Input: part model. Units: mm. Frame: model coordinates. A direction names the side the tool comes from. Coordinates: 2 decimals unless noted, no trailing zeros. Write each loop counter-clockwise with the first axis right and the second up, starting at its lowest first coordinate (ties: lowest second). Pieces come first, ordered by that corner, then holes.
1) Section query C-C (y = 6.5). Output: boundary loops of the cut face in (x, z).
2) Pin query (flat end, axial travel): pin 1 Ø5 at (x, y) = (0, 7) entering from -Z; pin 2 Ø2 at (y, z) = (2.5, -8) entering from -X; pin 3 Ø5 at (y, z) = (3, -4) entering from -X; pin 4 Ø5 at (x, y) = (9.5, 7) entering from -Z. Return the tip coordinate at first contact, or that it passes through.
3) Section query B-B (z = 0). Output: boundary loops of the cut face in (x, y).
4) Set-up query: faces 1 (the cylindrical face through (-2.75, 1.9, 12.4)), 2 (the cylindrical face through (-1.38, 5.67, 6.2)). Return all of +Z, -Z, +X, -X, +Y, -Y with unobstructed straight access to the full face (end or side cutting, diameter ignored); none if empty.
5) Section query A-A (x = 0). Output: boundary loops of the cut face in (y, z).
6) Line query: L1, parallel to Y at x = 3.25, z = 6.25; L2, parallel to Z at x = 3, y = 1.25; L3, parallel to Z at x = -4.75, y = 2.5. Output: solid intervals per line, ascending.
from build123d import *

# Parameters (mm, degrees)
SKETCH1_R           = 12.7
BOSS_EXTRUDE1_DEPTH = 2.54
SKETCH2_R           = 6.35
BOSS_EXTRUDE2_DEPTH = 6.35
CHAMFER1_SIZE       = 1.27


with BuildPart() as part:
    # Sketch1 → Boss-Extrude1 (new body)
    with BuildSketch(Plane(origin=(0, 0, 0), x_dir=(1, 0, 0), z_dir=(0, 1, 0))):
        Circle(SKETCH1_R)
    extrude(amount=BOSS_EXTRUDE1_DEPTH)

    # Sketch2 → Boss-Extrude2 (add)
    with BuildSketch(Plane(origin=(0, 2.54, 0), x_dir=(1, 0, 0), z_dir=(0, 1, 0))):
        Circle(SKETCH2_R)
    extrude(amount=BOSS_EXTRUDE2_DEPTH)

    # Chamfer1
    chamfer1_edges = [part.edges().sort_by_distance(p)[0] for p in [
        (-12.7, 0, 0),
    ]]
    chamfer(chamfer1_edges, length=CHAMFER1_SIZE)


solid = part.part
Answer:
1. outline: circle Ø12.7 at (0, 0)
2. pin 1: stops at z = -6.35
2. pin 2: stops at x = -10.6
2. pin 3: stops at x = -12.61
2. pin 4: passes through
3. outline: (-12.7, 1.27) - (-11.43, 0) - (11.43, 0) - (12.7, 1.27) - (12.7, 2.54) - (6.35, 2.54) - (6.35, 8.89) - (-6.35, 8.89) - (-6.35, 2.54) - (-12.7, 2.54) - close
4. face 1: +Y, -Y
4. face 2: +Y
5. outline: (0, -11.43) - (1.27, -12.7) - (2.54, -12.7) - (2.54, -6.35) - (8.89, -6.35) - (8.89, 6.35) - (2.54, 6.35) - (2.54, 12.7) - (1.27, 12.7) - (0, 11.43) - close
6. L1: y = 0 to 2.54
6. L2: z = -12.32 to 12.32
6. L3: z = -11.78 to 11.78
